Geometry check sheet. Reference: the model listing, model coordinates, mm. A direction names the side the tool comes from. Coordinates: 2 decimals unless noted, no trailing zeros. Write each loop counter-clockwise with the first axis right and the second up, starting at its lowest first coordinate (ties: lowest second). Pieces come first, ordered by that corner, then holes.
from build123d import *

# Parameters (mm, degrees)
BOSS_EXTRUDE1_DEPTH      = 76.2
BOSS_EXTRUDE1_DEPTH_BACK = 25.4
SKETCH1_W                = 2704.084
SKETCH1_H                = 1152.398
SKETCH1_W_2              = 387.096
SKETCH1_H_2              = 129.032
SKETCH2_R                = 76.2
CUT_EXTRUDE1_DEPTH       = 76.2
FILLET1_R                = 2.54


with BuildPart() as part:
    # Sketch1 → Boss-Extrude1 (new, two sides: drawn at the far end of the back side and taken through both)
    with BuildSketch(Plane.XY.offset(-BOSS_EXTRUDE1_DEPTH_BACK)):
        with Locations((1352.042, 576.199)):
            Rectangle(SKETCH1_W, SKETCH1_H)
        with Locations((1355.344, 1011.682)):
            Rectangle(SKETCH1_W_2, SKETCH1_H_2, mode=Mode.SUBTRACT)
    extrude(amount=BOSS_EXTRUDE1_DEPTH + BOSS_EXTRUDE1_DEPTH_BACK)

    # Sketch2 → Cut-Extrude1 (cut)
    with BuildSketch(Plane(origin=(2704.084, 0, 0), x_dir=(0, 0, -1), z_dir=(1, 0, 0))):
        with Locations((-76.2, 576.199)):
            Circle(SKETCH2_R)
    extrude(amount=-CUT_EXTRUDE1_DEPTH, mode=Mode.SUBTRACT)

    # Fillet1
    fillet1_edges = [part.edges().sort_by_distance(p)[0] for p in [
        (2704.084, 576.199, -25.4),
        (1352.042, 1152.398, -25.4),
        (0, 576.199, -25.4),
        (0, 1152.398, 25.4),
        (2704.084, 1152.398, 25.4),
        (2704.084, 0, 25.4),
        (0, 0, 25.4),
        (1352.042, 0, -25.4),
    ]]
    fillet(fillet1_edges, radius=FILLET1_R)


solid = part.part
1. Sectioned sample at C-C, the plane y = 588.5. Record the boundary of the cut face in (x, z).
Computed values:
outline: (0, -22.86) arc R2.54 ccw to (2.54, -25.4) - (2701.54, -25.4) arc R2.54 ccw to (2704.08, -22.86) - (2704.08, 1) - (2627.88, 1) - (2627.88, 76.2) - (0, 76.2) - close
2. Thickness scan on line 1 along X through (y, z) = (1019.5, 37); line 2 along X through (y, z) = (573, 60). Record the ranges inside material, lowest first.
Computed values:
line 1: x = 0 to 1161.8, 1548.89 to 2704.08
line 2: x = 0 to 2627.88
3. Sectioned sample at A-A, the plane x = 1228.5. Record the boundary of the cut face in (y, z), and give its area (3 significant figures).
Computed values:
outline: (0, -22.86) arc R2.54 ccw to (2.54, -25.4) - (947.17, -25.4) - (947.17, 76.2) - (0, 76.2) - close; (1076.2, -25.4) - (1149.86, -25.4) arc R2.54 ccw to (1152.4, -22.86) - (1152.4, 76.2) - (1076.2, 76.2) - close
area: 104,000 mm2
4. Sectioned sample at B-B, the plane z = 39. Record the boundary of the cut face in (x, y).
Computed values:
outline: (0, 2.54) arc R2.54 ccw to (2.54, 0) - (2701.54, 0) arc R2.54 ccw to (2704.08, 2.54) - (2704.08, 509.7) - (2627.88, 509.7) - (2627.88, 642.7) - (2704.08, 642.7) - (2704.08, 1149.86) arc R2.54 ccw to (2701.54, 1152.4) - (2.54, 1152.4) arc R2.54 ccw to (0, 1149.86) - close; hole (1161.8, 947.17) - (1548.89, 947.17) - (1548.89, 1076.2) - (1161.8, 1076.2) - close
5. Gauge pin test, flat end, axial feed: pin 1 Ø1.5 at (y, z) = (534.5, 63.5) entering from +X. Record the tip position at first contact, or that the pin passes through.
Computed values:
pin 1: stops at x = 2627.88
6. Access from +Z, -Z, +X, -X, +Y, -Y to the whole of each face (thin tool, end or side, straight path). Record for faces 1 (the flat face through (1333, 1152.398, 26)), 2 (the flat face through (1353, 947.166, 25)), 3 (the cylindrical face through (2666.52, 574.52, 0.02)).
Computed values:
face 1: +Z, -Z, +X, -X, +Y
face 2: +Z, -Z
face 3: +Z, +X
7. Draft check along X on faces 4 (the flat face through (2704.084, 568, -7)), 5 (the flat face through (1548.892, 1011, 25)), 6 (the flat face through (1333, 584, 76.2)). Enter one of: released by +X, released by -X, zero draft, split by the parting line, or undercut.
Computed values:
face 4: released by +X
face 5: undercut
face 6: zero draft
